Design review of the part built by this model. Coordinates are the model's own, in mm. A direction names the side the tool comes from. Coordinates: 2 decimals unless noted, no trailing zeros. Loops run counter-clockwise (first coordinate to the right, second up) from the corner with the lowest first, then second, coordinate; pieces in that order, holes last.
Q1. Add section A-A on z = 51. Give the boundary of the cut face in (x, y), and give its area (3 significant figures).
Q2. For P1, Ø2, axis at x = 4, z = -5, coming from the -Y side; P2, Ø5, axis at y = -3.5, z = 57.5, coming from the +X side; P3, Ø6, axis at y = 4.5, z = 74.5, coming from the -X side, all flat-tipped, find the tip position at first contact; note any pin that passes through.
Q3. Wall thickness on probe 1 along X at (y, z) = (0, 38.5); probe 2 along X at (y, z) = (1, -30): over which ranges is each line inside the solid? List them lowest first.
Q4. Draft analysis for pull direction X (two halves, no side actions). For faces 1 (the face through (0, -2, -1)), 2 (the face through (2.2, 0.1, -100)), 3 (the face through (-6, 0, 72)), state which applies: released by +X, released by -X, zero draft, split by the parting line, or undercut.
Q5. Machinability: for faces 4 (the face through (-1.301, -5.857, -2.471)), 5 (the face through (-3.09, 4.85, 43.96)), which of the approach directions +Z, -Z, +X, -X, +Y, -Y give a long, thin tool a straight path to every point of the face, cutting with its end or side? Answer none if there is none.
```python
from build123d import *

# Parameters (mm, degrees)
SKETCH1_R           = 6
EXTRUDE1_DEPTH      = 100
CHAMFER1_SIZE       = 0.9
EXTRUDE3_DEPTH      = 101.359354322
EXTRUDE3_DEPTH_BACK = 101.359354322
SKETCH2_R           = 2


with BuildPart() as part:
    # Sketch1 → Extrude1 (new, symmetric)
    with BuildSketch(Plane.XY):
        Circle(SKETCH1_R)
    extrude(amount=EXTRUDE1_DEPTH, both=True)

    # Chamfer1
    chamfer1_edges = [part.edges().sort_by_distance(p)[0] for p in [
        (-6, 0, -100),
        (-6, 0, 100),
    ]]
    chamfer(chamfer1_edges, length=CHAMFER1_SIZE)

    # Sketch2 → Extrude3 (cut, two sides: drawn at the far end of the back side and taken through both)
    with BuildSketch(Plane.XY.offset(-EXTRUDE3_DEPTH_BACK)):
        Circle(SKETCH2_R)
    extrude(amount=EXTRUDE3_DEPTH + EXTRUDE3_DEPTH_BACK, mode=Mode.SUBTRACT)

    # Sketch5 → Groove for DIN 471 - 12 x 1_ Circlip for (revolve, cut)
    with BuildSketch(Plane(origin=(0, 0, 100), x_dir=(0, 1, 0), z_dir=(-1, 0, 0)), mode=Mode.PRIVATE) as groove_for_din_471_12_x_1_circlip_for_sk:
        with BuildLine():
            Line((5.86, 55.5), (7.2, 55.5))
            Line((7.2, 55.5), (7.2, 56.6))
            Line((7.2, 56.6), (5.86, 56.6))
            ThreePointArc((5.86, 56.6), (5.782218254, 56.567781746), (5.75, 56.49))
            Line((5.75, 56.49), (5.75, 55.61))
            ThreePointArc((5.75, 55.61), (5.782218254, 55.532218254), (5.86, 55.5))
        make_face()
    revolve(groove_for_din_471_12_x_1_circlip_for_sk.sketch.rotate(Axis((0, 0, 150), (0, 0, -1)), 270), axis=Axis((0, 0, 150), (0, 0, -1)), mode=Mode.SUBTRACT)

    # Sketch7 → Groove for DIN 471 - 12 x 1_ Circlip 2 (revolve, cut)
    with BuildSketch(Plane(origin=(0, 0, 100), x_dir=(0, 1, 0), z_dir=(-1, 0, 0)), mode=Mode.PRIVATE) as groove_for_din_471_12_x_1_circlip_2_sk:
        with BuildLine():
            Line((5.899017031, 149.607152194), (7.198150102, 150.1))
            Line((7.198150102, 150.1), (7.2, 150.7))
            Line((7.2, 150.7), (5.86, 150.7))
            ThreePointArc((5.86, 150.7), (5.782218254, 150.667781746), (5.75, 150.59))
            Line((5.75, 150.59), (5.75, 149.71))
            ThreePointArc((5.75, 149.71), (5.797517496, 149.619468587), (5.899017031, 149.607152194))
        make_face()
    revolve(groove_for_din_471_12_x_1_circlip_2_sk.sketch.rotate(Axis((0, 0, 150), (0, 0, -1)), 270), axis=Axis((0, 0, 150), (0, 0, -1)), mode=Mode.SUBTRACT)


solid = part.part
```
Entries:
1. outline: circle Ø12 at (0, 0); hole circle Ø4 at (0, 0)
1. area: 101 mm2
2. P1: stops at y = -5.2
2. P2: stops at x = 5.92
2. P3: stops at x = -5.81
3. probe 1: x = -6 to -2, 2 to 6
3. probe 2: x = -5.92 to -1.73, 1.73 to 5.92
4. face 1: undercut
4. face 2: zero draft
4. face 3: split by the parting line
5. face 4: +Z, -Z
5. face 5: none
